Read the model definition and answer for the solid it produces. Units are mm, in the model's axes. A direction names the side the tool comes from. Give positions to 0.01 mm unless a question says otherwise; leave off trailing zeros. Write each loop counter-clockwise with the first axis right and the second up, starting at its lowest first coordinate (ties: lowest second). Pieces come first, ordered by that corner, then holes. Notation, with made-up numbers: (64, 49.5) - (96, 49.5) arc R38 ccw to (96, 87.5) - close; hole circle Ø10 at (11.5, -26.5). An arc over 180 degrees is marked (long way). Use CSV: the item, a comma, the result in double quotes. Start each with the question number.
from build123d import *

# Parameters (mm, degrees)
F1_DEPTH = 12.5
F2_R     = 5
F3_SIZE  = 2
F4_R     = 5


with BuildPart() as f1:
    # F0 (on Front) → F1 (new body, symmetric)
    with BuildSketch(Plane.XZ):
        with BuildLine():
            Line((-41.361794, 112.736205), (-40.251029, 91.541546))
            ThreePointArc((-40.251029, 91.541546), (-45.39905, 89.100652), (-50.399706, 86.370537))
            Line((-50.399706, 86.370537), (-66.893654, 99.727073))
            Line((-66.893654, 99.727073), (-70.53423, 97.082039))
            Line((-70.53423, 97.082039), (-74.174807, 94.437006))
            Line((-74.174807, 94.437006), (-66.568897, 74.622932))
            ThreePointArc((-66.568897, 74.622932), (-70.710678, 70.710678), (-74.622932, 66.568897))
            Line((-74.622932, 66.568897), (-94.437006, 74.174807))
            Line((-94.437006, 74.174807), (-97.082039, 70.53423))
            Line((-97.082039, 70.53423), (-99.727073, 66.893654))
            Line((-99.727073, 66.893654), (-86.370537, 50.399706))
            ThreePointArc((-86.370537, 50.399706), (-89.100652, 45.39905), (-91.541546, 40.251029))
            Line((-91.541546, 40.251029), (-112.736205, 41.361794))
            Line((-112.736205, 41.361794), (-114.126782, 37.082039))
            Line((-114.126782, 37.082039), (-115.517358, 32.802285))
            Line((-115.517358, 32.802285), (-97.717628, 21.243005))
            ThreePointArc((-97.717628, 21.243005), (-98.768834, 15.643447), (-99.499436, 9.99311))
            Line((-99.499436, 9.99311), (-120, 4.5))
            Line((-120, 4.5), (-120, 0))
            Line((-120, 0), (-120, -4.5))
            Line((-120, -4.5), (-99.499436, -9.99311))
            ThreePointArc((-99.499436, -9.99311), (-98.768834, -15.643447), (-97.717628, -21.243005))
            Line((-97.717628, -21.243005), (-115.517358, -32.802285))
            Line((-115.517358, -32.802285), (-114.126782, -37.082039))
            Line((-114.126782, -37.082039), (-112.736205, -41.361794))
            Line((-112.736205, -41.361794), (-91.541546, -40.251029))
            ThreePointArc((-91.541546, -40.251029), (-89.100652, -45.39905), (-86.370537, -50.399706))
            Line((-86.370537, -50.399706), (-99.727073, -66.893654))
            Line((-99.727073, -66.893654), (-97.082039, -70.53423))
            Line((-97.082039, -70.53423), (-94.437006, -74.174807))
            Line((-94.437006, -74.174807), (-74.622932, -66.568897))
            ThreePointArc((-74.622932, -66.568897), (-70.710678, -70.710678), (-66.568897, -74.622932))
            Line((-66.568897, -74.622932), (-74.174807, -94.437006))
            Line((-74.174807, -94.437006), (-70.53423, -97.082039))
            Line((-70.53423, -97.082039), (-66.893654, -99.727073))
            Line((-66.893654, -99.727073), (-50.399706, -86.370537))
            ThreePointArc((-50.399706, -86.370537), (-45.39905, -89.100652), (-40.251029, -91.541546))
            Line((-40.251029, -91.541546), (-41.361794, -112.736205))
            Line((-41.361794, -112.736205), (-37.082039, -114.126782))
            Line((-37.082039, -114.126782), (-32.802285, -115.517358))
            Line((-32.802285, -115.517358), (-21.243005, -97.717628))
            ThreePointArc((-21.243005, -97.717628), (-15.643447, -98.768834), (-9.99311, -99.499436))
            Line((-9.99311, -99.499436), (-4.5, -120))
            Line((-4.5, -120), (0, -120))
            Line((0, -120), (4.5, -120))
            Line((4.5, -120), (9.99311, -99.499436))
            ThreePointArc((9.99311, -99.499436), (15.643447, -98.768834), (21.243005, -97.717628))
            Line((21.243005, -97.717628), (32.802285, -115.517358))
            Line((32.802285, -115.517358), (37.082039, -114.126782))
            Line((37.082039, -114.126782), (41.361794, -112.736205))
            Line((41.361794, -112.736205), (40.251029, -91.541546))
            ThreePointArc((40.251029, -91.541546), (45.39905, -89.100652), (50.399706, -86.370537))
            Line((50.399706, -86.370537), (66.893654, -99.727073))
            Line((66.893654, -99.727073), (70.53423, -97.082039))
            Line((70.53423, -97.082039), (74.174807, -94.437006))
            Line((74.174807, -94.437006), (66.568897, -74.622932))
            ThreePointArc((66.568897, -74.622932), (70.710678, -70.710678), (74.622932, -66.568897))
            Line((74.622932, -66.568897), (94.437006, -74.174807))
            Line((94.437006, -74.174807), (97.082039, -70.53423))
            Line((97.082039, -70.53423), (99.727073, -66.893654))
            Line((99.727073, -66.893654), (86.370537, -50.399706))
            ThreePointArc((86.370537, -50.399706), (89.100652, -45.39905), (91.541546, -40.251029))
            Line((91.541546, -40.251029), (112.736205, -41.361794))
            Line((112.736205, -41.361794), (114.126782, -37.082039))
            Line((114.126782, -37.082039), (115.517358, -32.802285))
            Line((115.517358, -32.802285), (97.717628, -21.243005))
            ThreePointArc((97.717628, -21.243005), (98.768834, -15.643447), (99.499436, -9.99311))
            Line((99.499436, -9.99311), (120, -4.5))
            Line((120, -4.5), (120, 0))
            Line((120, 0), (120, 4.5))
            Line((120, 4.5), (99.499436, 9.99311))
            ThreePointArc((99.499436, 9.99311), (98.768834, 15.643447), (97.717628, 21.243005))
            Line((97.717628, 21.243005), (115.517358, 32.802285))
            Line((115.517358, 32.802285), (114.126782, 37.082039))
            Line((114.126782, 37.082039), (112.736205, 41.361794))
            Line((112.736205, 41.361794), (91.541546, 40.251029))
            ThreePointArc((91.541546, 40.251029), (89.100652, 45.39905), (86.370537, 50.399706))
            Line((86.370537, 50.399706), (99.727073, 66.893654))
            Line((99.727073, 66.893654), (97.082039, 70.53423))
            Line((97.082039, 70.53423), (94.437006, 74.174807))
            Line((94.437006, 74.174807), (74.622932, 66.568897))
            ThreePointArc((74.622932, 66.568897), (70.710678, 70.710678), (66.568897, 74.622932))
            Line((66.568897, 74.622932), (74.174807, 94.437006))
            Line((74.174807, 94.437006), (70.53423, 97.082039))
            Line((70.53423, 97.082039), (66.893654, 99.727073))
            Line((66.893654, 99.727073), (50.399706, 86.370537))
            ThreePointArc((50.399706, 86.370537), (45.39905, 89.100652), (40.251029, 91.541546))
            Line((40.251029, 91.541546), (41.361794, 112.736205))
            Line((41.361794, 112.736205), (37.082039, 114.126782))
            Line((37.082039, 114.126782), (32.802285, 115.517358))
            Line((32.802285, 115.517358), (21.243005, 97.717628))
            ThreePointArc((21.243005, 97.717628), (15.643447, 98.768834), (9.99311, 99.499436))
            Line((9.99311, 99.499436), (4.5, 120))
            Line((4.5, 120), (0, 120))
            Line((0, 120), (-4.5, 120))
            Line((-4.5, 120), (-9.99311, 99.499436))
            ThreePointArc((-9.99311, 99.499436), (-15.643447, 98.768834), (-21.243005, 97.717628))
            Line((-21.243005, 97.717628), (-32.802285, 115.517358))
            Line((-32.802285, 115.517358), (-37.082039, 114.126782))
            Line((-37.082039, 114.126782), (-41.361794, 112.736205))
        make_face()
    extrude(amount=F1_DEPTH, both=True)

    # F2
    f2_edges = [f1.edges().sort_by_distance(p)[0] for p in [
        (40.251029, 0, 91.541546),
        (50.399706, 0, 86.370537),
    ]]
    fillet(f2_edges, radius=F2_R)

    # F3
    f3_edges = [f1.edges().sort_by_distance(p)[0] for p in [
        (-66.893654, 0, 99.727073),
        (-74.174807, 0, 94.437006),
        (-32.802285, 0, 115.517358),
        (-41.361794, 0, 112.736205),
        (4.5, 0, 120),
        (-4.5, 0, 120),
        (41.361794, 0, 112.736205),
        (32.802285, 0, 115.517358),
        (74.174807, 0, 94.437006),
        (66.893654, 0, 99.727073),
        (99.727073, 0, 66.893654),
        (94.437006, 0, 74.174807),
        (115.517358, 0, 32.802285),
        (112.736205, 0, 41.361794),
        (120, 0, -4.5),
        (120, 0, 4.5),
        (112.736205, 0, -41.361794),
        (115.517358, 0, -32.802285),
        (94.437006, 0, -74.174807),
        (99.727073, 0, -66.893654),
        (66.893654, 0, -99.727073),
        (74.174807, 0, -94.437006),
        (32.802285, 0, -115.517358),
        (41.361794, 0, -112.736205),
        (-4.5, 0, -120),
        (4.5, 0, -120),
        (-41.361794, 0, -112.736205),
        (-32.802285, 0, -115.517358),
        (-74.174807, 0, -94.437006),
        (-66.893654, 0, -99.727073),
        (-99.727073, 0, -66.893654),
        (-94.437006, 0, -74.174807),
        (-112.736205, 0, -41.361794),
        (-115.517358, 0, -32.802285),
        (-120, 0, -4.5),
        (-120, 0, 4.5),
        (-115.517358, 0, 32.802285),
        (-112.736205, 0, 41.361794),
        (-99.727073, 0, 66.893654),
        (-94.437006, 0, 74.174807),
    ]]
    chamfer(f3_edges, length=F3_SIZE)

    # F4
    f4_edges = [f1.edges().sort_by_distance(p)[0] for p in [
        (74.622932, 0, 66.568897),
        (66.568897, 0, 74.622932),
        (91.541546, 0, 40.251029),
        (86.370537, 0, 50.399706),
        (97.717628, 0, 21.243005),
        (99.499436, 0, 9.99311),
        (99.499436, 0, -9.99311),
        (97.717628, 0, -21.243005),
        (91.541546, 0, -40.251029),
        (86.370537, 0, -50.399706),
    ]]
    fillet(f4_edges, radius=F4_R)


solid = f1.part
(1) For a pull along X with two mould halves and no side action, classify faces 1 (the face through (-2, -12.5, 2)), 2 (the face through (-40.76, -0.18, 101.27)), 3 (the face through (-105.89, -0.18, 26.55)), 4 (the face through (70.582, -0.175, 85.076)) as pulls with the +X half, pulls with the -X half, needs draft (parallel to the pull), parting line crosses it, or undercut.
(2) Consider probe 1 along X at (y, z) = (-6.5, -107.5); probe 2 along Z at (x, y) = (-66.5, 9.75); probe 3 along Z at (x, y) = (65, -8.75). Determine where each line is inside the solid, lowest interval first.
(3) The part is cut by section B-B on z = 82. Write down the section's boundary in (x, y).
(4) Given P1, Ø1, axis at y = 6, z = 68, coming from the -X side; P2, Ø2, axis at x = 87.5, y = -5, coming from the +Z side; P3, Ø2, axis at y = -5.5, z = 95.5, coming from the -X side, each flat-ended and moving along its own axis, determine where each tip first touches the part or whether it passes through.
(5) The part is cut by section A-A on x = 105.5. Write down the section's boundary in (y, z).
(6) Which of the six approach directions +Z, -Z, +X, -X, +Y, -Y give full straight-line access (tool end or side, diameter ignored) to faces 5 (the face through (-108.91, -0.18, -7.47)), 6 (the face through (110.529, -0.175, 7.038)), 7 (the face through (-101.006, -0.175, 40.747)), 8 (the face through (-83.72, -0.18, -70.06))?
(7) The part is cut by section C-C on x = 61. Write down the section's boundary in (y, z).
Reported:
1,face 1,"needs draft"
1,face 2,"undercut"
1,face 3,"pulls with the -X half"
1,face 4,"pulls with the +X half"
2,probe 1,"-41.09 to -27.6, -7.85 to 7.85, 27.6 to 41.09"
2,probe 2,"-98.5 to 98.5"
2,probe 3,"-98.19 to 98.19"
3,outline,"(-69.4, -12.5) - (69.4, -12.5) - (69.4, 12.5) - (-69.4, 12.5) - close"
4,P1,"x = -98.55"
4,P2,"z = 71.9"
4,P3,"x = -72.89"
5,outline,"(-12.5, -40.98) - (12.5, -40.98) - (12.5, -26.3) - (-12.5, -26.3) - close; (-12.5, -8.39) - (12.5, -8.39) - (12.5, 8.39) - (-12.5, 8.39) - close; (-12.5, 26.3) - (12.5, 26.3) - (12.5, 40.98) - (-12.5, 40.98) - close"
6,face 5,"-X, +Y, -Y"
6,face 6,"+X, +Y, -Y"
6,face 7,"+Y, -Y"
6,face 8,"-Z, +Y, -Y"
7,outline,"(-12.5, -94.95) - (12.5, -94.95) - (12.5, 94.95) - (-12.5, 94.95) - close"
